Input: dimensioned drawing with shaded views. Units: mm. Origin: part minimum x, y, z. A direction names the side the tool comes from. Coordinates: 2 decimals unless noted, no trailing zeros. Order: outer loops, then holes, each group sorted by start corner. A loop starts at its lowest first (then second) coordinate and runs counter-clockwise, first axis right, second up. Notation, with made-up numbers: (86.5, 19) -> (141.5, 19) arc R22 cw to (141.5, 55) -> close; hole circle Ø10 at (40, -31.5). An arc over 180 degrees is marked (long way). Put each result on its own line as item: value.
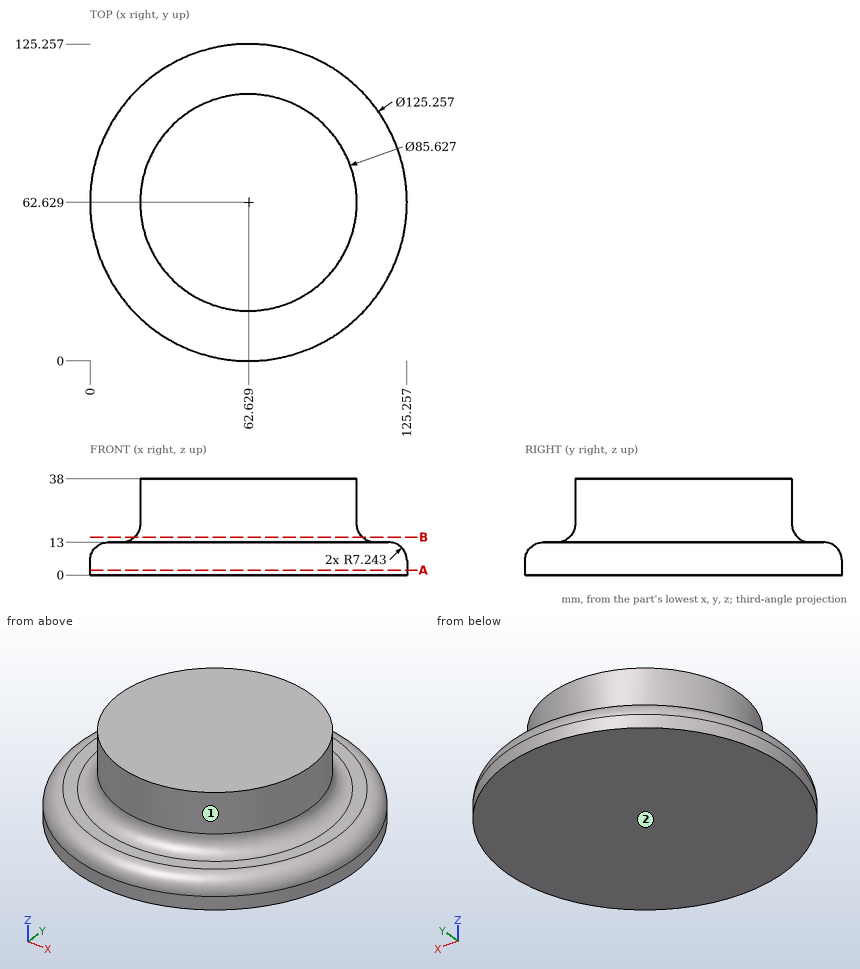
1. Cut plane B-B on z = 15. Output: boundary loops of the cut face in (x, y), plus the area to 3 significant figures.
Numbers:
outline: circle Ø90.12 at (62.63, 62.63)
area: 6,380 mm2
2. Ray query, line 1 along X through (y, z) = (25, 3) (1 decimal); line 2 along X through (y, z) = (63, 27.5); line 3 along Y through (x, z) = (45.5, 6.5). Return the intervals inside material, ascending.
Numbers:
line 1: x = 12.6 to 112.7
line 2: x = 19.82 to 105.44
line 3: y = 2.43 to 122.83
3. First-contact query: pin 1 (8 mm diameter, centred on x = 36.5, y = 103.5, fed in from +Z) (1 decimal); pin 2 (12 mm diameter, centred on y = 83, z = 28, fed in from -X); pin 3 (8 mm diameter, centred on x = 61, z = 24, fed in from +Y). Flat tips, straight axial feed; report the tip coordinate or a pass-through.
Numbers:
pin 1: stops at z = 15.6
pin 2: stops at x = 22.3
pin 3: stops at y = 105.44
4. Set-up query: the marked faces 1 and 2. Return all of +Z, -Z, +X, -X, +Y, -Y with unobstructed straight access to the full face (end or side cutting, diameter ignored); none if empty.
Numbers:
face 1: +Z
face 2: -Z, +X, -X, +Y, -Y
5. Cut plane A-A on z = 2. Output: boundary loops of the cut face in (x, y).
Numbers:
outline: circle Ø125.26 at (62.63, 62.63)
